Geometry: final body of the model. Coordinates: model frame, mm. A direction names the side the tool comes from. Give positions to 0.01 mm unless a question says otherwise; leave off trailing zeros. Loops run counter-clockwise (first coordinate to the right, second up) from the corner with the lowest first, then second, coordinate; pieces in that order, holes last. Notation, with made-up numbers: (55, -14) -> (83, -14) arc R25 cw to (83, 6) -> close; hole circle Ø3 at (74, -37). An arc over 180 degrees is marked (long way). Answer in a Markdown table with one row per item. Add a question column.
1) First-contact query: P1, Ø4, axis at x = 6, y = 18, coming from the -Z side; P2, Ø1.5, axis at y = 16, z = 4.5, coming from the +X side; P3, Ø1, axis at x = 19.5, z = 5.5, coming from the -Y side. Flat tips, straight axial feed; report the tip coordinate or a pass-through.
2) Section query B-B (x = 6). Return the cut outline in (y, z).
3) Draft query along Y for faces 3 (the flat face through (13, 48, 3)), 4 (the flat face through (7, 30, 6)), 5 (the cylindrical face through (5.74, 19.17, 2.96)). Return one class per face: +Y half, -Y half, draft (parallel to the pull), parting line (faces both ways), or undercut.
4) Line query: line 1 (Y direction, x = 6, z = 2.5); line 2 (X direction, y = 36.5, z = 0.35); line 3 (Y direction, x = 22, z = 2.45). Output: solid intervals per line, ascending. Write a range as from..to.
5) Section query D-D (y = 23). Return the cut outline in (x, z).
6) Section query A-A (y = 18). Return the cut outline in (x, z), plus the area to 3 significant figures.
7) Section query C-C (z = 3.9). Return the cut outline in (x, y).
8) Access query for faces 1 (the cylindrical face through (5.84, 6.81, 2.96)), 2 (the flat face through (18, 40, 3)). Directions: +Z, -Z, +X, -X, +Y, -Y. A direction counts if a zero-diameter tool reaches every point of the face in a straight line with its end or side. Return the directions, or none.
Solid Edge part; units mm, degrees
sketch "Sketch1" plane through (0, 0, 0) normal (0, 0, 1) x (1, 0, 0)
  line L0 (0, 0) -> (12, 0)
  line L1 (12, 0) -> (12, 40)
  line L2 (12, 40) -> (25, 40)
  line L3 (25, 40) -> (25, 48)
  line L4 (25, 48) -> (0, 48)
  line L5 (0, 48) -> (0, 0)
  circle A0 centre (6, 8) radius 1.2
  circle A1 centre (6, 18) radius 1.2
extrude "Protrusion1" add sketch "Sketch1" along normal blind 6
Evaluation:
| question | item | result |
|---|---|---|
| 1 | P1 | z = 0 |
| 1 | P2 | x = 12 |
| 1 | P3 | y = 40 |
| 2 | outline | (0, 0) -> (6.8, 0) -> (6.8, 6) -> (0, 6) -> close; (9.2, 0) -> (16.8, 0) -> (16.8, 6) -> (9.2, 6) -> close; (19.2, 0) -> (48, 0) -> (48, 6) -> (19.2, 6) -> close |
| 3 | face 3 | +Y half |
| 3 | face 4 | draft |
| 3 | face 5 | undercut |
| 4 | line 1 | 0..6.8, 9.2..16.8, 19.2..48 |
| 4 | line 2 | 0..12 |
| 4 | line 3 | 40..48 |
| 5 | outline | (0, 0) -> (12, 0) -> (12, 6) -> (0, 6) -> close |
| 6 | outline | (0, 0) -> (4.8, 0) -> (4.8, 6) -> (0, 6) -> close; (7.2, 0) -> (12, 0) -> (12, 6) -> (7.2, 6) -> close |
| 6 | area | 57.6 mm² |
| 7 | outline | (0, 0) -> (12, 0) -> (12, 40) -> (25, 40) -> (25, 48) -> (0, 48) -> close; hole circle Ø2.4 at (6, 8); hole circle Ø2.4 at (6, 18) |
| 8 | face 1 | +Z, -Z |
| 8 | face 2 | +Z, -Z, +X, -Y |
